from build123d import *

# Parameters (mm, degrees)
SKETCH2_R             = 15
BOSS_EXTRUDE5_DEPTH   = 40.513
SKETCH2_R_2           = 7.343075537
BOSS_EXTRUDE5_2_DEPTH = 40.513
SKETCH2_R_3           = 7.048050761
BOSS_EXTRUDE5_3_DEPTH = 40.513
SKETCH2_R_4           = 7.405031705
BOSS_EXTRUDE5_4_DEPTH = 40.513
BOSS_EXTRUDE6_DEPTH   = 4.7625
SKETCH9_R             = 1.27
CUT_EXTRUDE2_DEPTH    = 9.525
SKETCH10_R            = 4
BOSS_EXTRUDE7_DEPTH   = 28.575


with BuildPart() as part:
    # Sketch2 → Boss-Extrude5 (new, symmetric)
    with BuildSketch(Plane.XY):
        with Locations((-135.989964622, 14.806967819)):
            Circle(SKETCH2_R)
    extrude(amount=BOSS_EXTRUDE5_DEPTH, both=True)



with BuildPart() as body_2:
    # Sketch2 → Boss-Extrude5 2 (new, symmetric)
    with BuildSketch(Plane.XY):
        with Locations((-76.175726851, -35.218198752)):
            Circle(SKETCH2_R_2)
    extrude(amount=BOSS_EXTRUDE5_2_DEPTH, both=True)


with BuildPart() as body_3:
    # Sketch2 → Boss-Extrude5 3 (new, symmetric)
    with BuildSketch(Plane.XY):
        with Locations((-53.236134933, -23.53725338)):
            Circle(SKETCH2_R_3)
    extrude(amount=BOSS_EXTRUDE5_3_DEPTH, both=True)


with BuildPart() as body_4:
    # Sketch2 → Boss-Extrude5 4 (new, symmetric)
    with BuildSketch(Plane.XY):
        with Locations((-2.84319901, 123.138021163)):
            Circle(SKETCH2_R_4)
    extrude(amount=BOSS_EXTRUDE5_4_DEPTH, both=True)


with BuildPart() as part_1:
    add(part.part)

    add(body_2.part)  # Boss-Extrude6 merges body 2

    add(body_3.part)  # Boss-Extrude6 merges body 3

    add(body_4.part)  # Boss-Extrude6 merges body 4
    # Sketch6 → Boss-Extrude6 (add, symmetric)
    with BuildSketch(Plane.XY.offset(40.513)):
        with BuildLine():
            Line((-144.43677034, 2.411344674), (-80.310762347, -41.286331891))
            ThreePointArc((-80.310762347, -41.286331891), (-76.600330476, -42.54898794), (-72.768932333, -41.723159126))
            Line((-72.768932333, -41.723159126), (-49.966216141, -29.780862162))
            ThreePointArc((-49.966216141, -29.780862162), (-47.894807622, -28.135648979), (-46.575803889, -25.842683907))
            Line((-46.575803889, -25.842683907), (4.15447513, 120.715821505))
            ThreePointArc((4.15447513, 120.715821505), (1.535064989, 129.110064273), (-7.258334859, 129.082856736))
            Line((-7.258334859, 129.082856736), (-144.43677034, 27.202590964))
            ThreePointArc((-144.43677034, 27.202590964), (-150.989964622, 14.806967819), (-144.43677034, 2.411344674))
        make_face()
    extrude(amount=BOSS_EXTRUDE6_DEPTH, both=True)

    # Sketch9 → Cut-Extrude2 (cut)
    with BuildSketch(Plane(origin=(0, 0, -40.513), x_dir=(-1, 0, 0), z_dir=(0, 0, -1))):
        with Locations((53.236134933, -23.53725338)):
            Circle(SKETCH9_R)
        with Locations((76.175726851, -35.218198752)):
            Circle(SKETCH9_R)
        with Locations((2.84319901, 123.138021163)):
            Circle(SKETCH9_R)
    extrude(amount=-CUT_EXTRUDE2_DEPTH, mode=Mode.SUBTRACT)

    # Sketch10 → Boss-Extrude7 (add)
    with BuildSketch(Plane(origin=(0, 0, -40.513), x_dir=(-1, 0, 0), z_dir=(0, 0, -1))):
        with Locations((135.989964622, 14.806967819)):
            Circle(SKETCH10_R)
    extrude(amount=BOSS_EXTRUDE7_DEPTH)


solid = part_1.part
Geometry check sheet. Reference: the model listing, model coordinates, mm. A direction names the side the tool comes from. Round coordinates to 2 decimals unless told otherwise and drop trailing zeros. Write each loop counter-clockwise with the first axis right and the second up, starting at its lowest first coordinate (ties: lowest second). Pieces come first, ordered by that corner, then holes. Notation, with made-up numbers: (-1, 27) -> (6, 27) arc R28 ccw to (6, 47) -> close; hole circle Ø4 at (21.25, 51). An arc over 180 degrees is marked (long way). One line per item, written item: value. Start each with the question number.
(1) Cross-section at D-D, the plane z = -22. Record the cut outline in (x, y).
(2) Cross-section at B-B, the plane x = -125. Record the cut outline in (y, z).
(3) Cross-section at C-C, the plane y = 25. Record the cut outline in (x, z).
(4) Go/stop test with flat-tipped pins: pin 1 Ø4.5 at (x, y) = (-73.5, -33.5) entering from -Z; pin 2 Ø1.3 at (x, y) = (-76.5, -35.5) entering from -Z; pin 3 Ø9 at (x, y) = (-136.5, 9) entering from -Z; pin 4 Ø4 at (y, z) = (19.5, -51.5) entering from -X. Record where each tip stops, or that it passes through.
(5) Cross-section at A-A, the plane z = -33.5. Record the cut outline in (x, y), and give its area (3 significant figures).
(6) Scan lines: line 1 (Z direction, x = -109, y = -3); line 2 (Y direction, x = -53, z = -10.5); line 3 (Y direction, x = -136, z = -1). Record each from-to range of solid material in increasing order. Write a range as [from, to].
(7) Access from +Z, -Z, +X, -X, +Y, -Y to the whole of each face (thin tool, end or side, straight path). Record for faces 1 (the flat face through (-132.9, 11.7, -40.513)), 2 (the flat face through (-53, -25, -40.513)).
Answer:
1. outline: circle Ø30 at (-135.99, 14.81); circle Ø14.69 at (-76.18, -35.22); circle Ø14.1 at (-53.24, -23.54); circle Ø14.81 at (-2.84, 123.14)
2. outline: (-10.83, 35.75) -> (4.6, 35.75) -> (4.6, -40.51) -> (25.02, -40.51) -> (25.02, 35.75) -> (41.64, 35.75) -> (41.64, 45.28) -> (-10.83, 45.28) -> close
3. outline: (-146.99, -40.51) -> (-124.99, -40.51) -> (-124.99, 35.75) -> (-28.98, 35.75) -> (-28.98, 45.28) -> (-146.99, 45.28) -> close
4. pin 1: z = -40.51
4. pin 2: z = -30.99
4. pin 3: z = -69.09
4. pin 4: x = -138.95
5. outline: circle Ø30 at (-135.99, 14.81); circle Ø14.69 at (-76.18, -35.22); circle Ø14.1 at (-53.24, -23.54); circle Ø14.81 at (-2.84, 123.14); hole circle Ø2.54 at (-76.18, -35.22); hole circle Ø2.54 at (-53.24, -23.54); hole circle Ø2.54 at (-2.84, 123.14)
5. area: 1,190 mm²
6. line 1: [35.75, 45.28]
6. line 2: [-30.58, -16.49]
6. line 3: [-0.19, 29.81]
7. face 1: -Z
7. face 2: -Z, +X, -X, +Y, -Y
